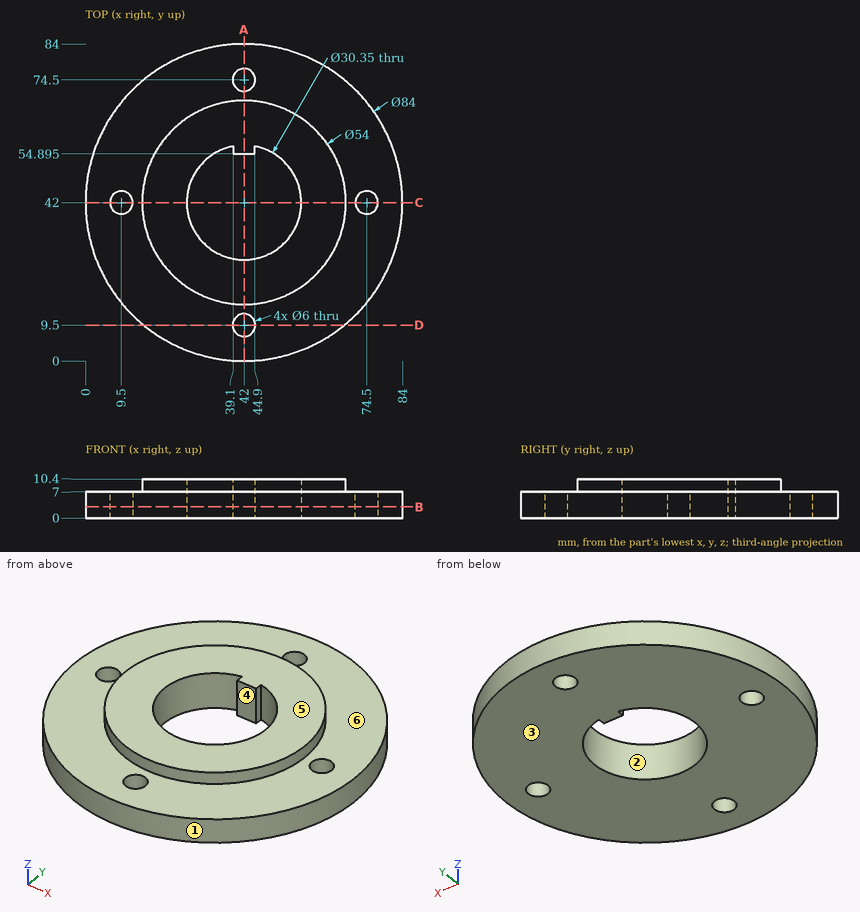
Input: dimensioned drawing with shaded views. Units: mm. Origin: part minimum x, y, z. A direction names the side the tool comes from. Coordinates: 2 decimals unless noted, no trailing zeros. Order: outer loops, then holes, each group sorted by start corner. A loop starts at its lowest first (then second) coordinate and runs counter-clockwise, first axis right, second up.
(1) Section query B-B (z = 3). State how many separate pieces and enclosed holes the cut face has, plus the area to 3 significant figures.
(2) Material intervals for probe 1 along X at (y, z) = (75, 2.75); probe 2 along X at (y, z) = (72, 0.75) (1 decimal); probe 3 along Z at (x, y) = (46.5, 73.5), sorted ascending.
(3) Section query D-D (y = 9.5). Return the cut outline in (x, z).
(4) Section query A-A (x = 42). Return the cut outline in (y, z) (1 decimal), plus the area to 3 significant figures.
(5) First-contact query: pin 1 (10 mm diameter, centred on x = 65.5, y = 69.5, fed in from -Z); pin 2 (6 mm diameter, centred on x = 74.5, z = 7, fed in from +Y) (1 decimal); pin 3 (0.6 mm diameter, centred on y = 56, z = 4.5, fed in from +X); pin 4 (1 mm diameter, centred on x = 41.5, y = 72, fed in from +Z). Flat tips, straight axial feed; report the tip coordinate or a pass-through.
(6) Draft query along Y for the marked faces 1, 2 and 3. Return one class per face: pulls with the +Y half, pulls with the -Y half, needs draft (parallel to the pull), parting line crosses it, or undercut.
(7) Section query C-C (y = 42). Return the cut outline in (x, z) (1 decimal), plus the area to 3 significant figures.
(8) Access query for the marked faces 4, 5 and 6. Directions: +Z, -Z, +X, -X, +Y, -Y. A direction counts if a zero-diameter tool reaches every point of the face in a straight line with its end or side. Return the directions, or none.
Solution:
1. separate pieces: 1
1. enclosed holes: 5
1. area: 4,720 mm2
2. probe 1: x = 16.02 to 39.04, 44.96 to 67.98
2. probe 2: x = 12.6 to 40.3, 43.7 to 71.4
2. probe 3: z = 0 to 7
3. outline: (15.4, 0) - (39, 0) - (39, 7) - (15.4, 7) - close; (45, 0) - (68.6, 0) - (68.6, 7) - (45, 7) - close
4. outline: (0, 0) - (6.5, 0) - (6.5, 7) - (0, 7) - close; (12.5, 0) - (26.8, 0) - (26.8, 10.4) - (15, 10.4) - (15, 7) - (12.5, 7) - close; (54.9, 0) - (71.5, 0) - (71.5, 7) - (69, 7) - (69, 10.4) - (54.9, 10.4) - close; (77.5, 0) - (84, 0) - (84, 7) - (77.5, 7) - close
4. area: 396 mm2
5. pin 1: stops at z = 0
5. pin 2: stops at y = 71.9
5. pin 3: stops at x = 81.7
5. pin 4: stops at z = 7
6. face 1: parting line crosses it
6. face 2: undercut
6. face 3: needs draft
7. outline: (0, 0) - (6.5, 0) - (6.5, 7) - (0, 7) - close; (12.5, 0) - (26.8, 0) - (26.8, 10.4) - (15, 10.4) - (15, 7) - (12.5, 7) - close; (57.2, 0) - (71.5, 0) - (71.5, 7) - (69, 7) - (69, 10.4) - (57.2, 10.4) - close; (77.5, 0) - (84, 0) - (84, 7) - (77.5, 7) - close
7. area: 372 mm2
8. face 4: +Z, -Z
8. face 5: +Z, +X, -X, +Y, -Y
8. face 6: +Z
